Geometry check sheet. Reference: drawing and pictorial views, mm from the part's lowest x, y, z. Coordinates: 2 decimals unless noted, no trailing zeros. Loops run counter-clockwise (first coordinate to the right, second up) from the corner with the lowest first, then second, coordinate; pieces in that order, holes last. Notation, with made-up numbers: (-31, 82) - (18, 82) arc R20 cw to (18, 117) - close; hole circle Ø10 at (-36.5, -10). An arc over 180 degrees is marked (long way). One line per item, written item: value.
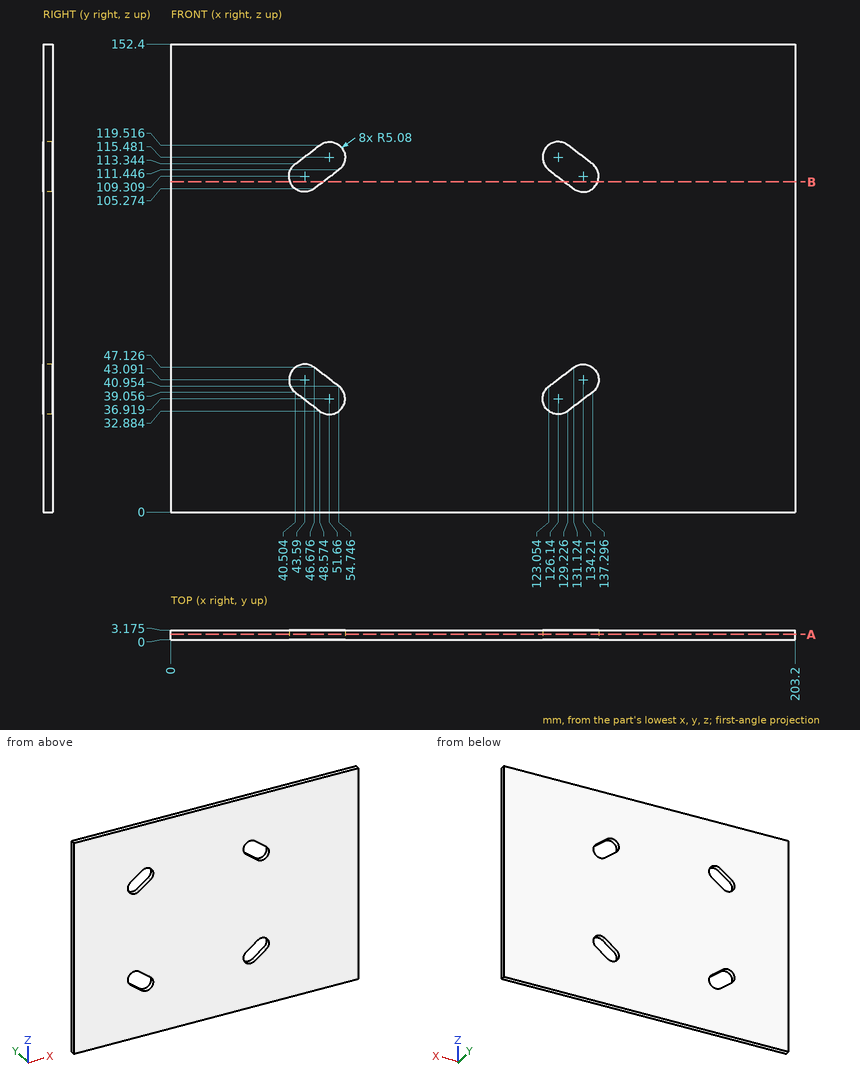
(1) Cross-section at A-A on y = 1.8. Record the cut outline in (x, z) (1 decimal), and give its area (3 significant figures).
Reply:
outline: (0, 0) - (203.2, 0) - (203.2, 152.4) - (0, 152.4) - close; hole (40.5, 39.1) - (48.6, 32.9) arc R5.1 ccw to (54.7, 41) - (46.7, 47.1) arc R5.1 ccw to start; hole (40.5, 113.3) arc R5.1 ccw to (46.7, 105.3) - (54.7, 111.4) arc R5.1 ccw to (48.6, 119.5) - close; hole (123.1, 41) arc R5.1 ccw to (129.2, 32.9) - (137.3, 39.1) arc R5.1 ccw to (131.1, 47.1) - close; hole (123.1, 111.4) - (131.1, 105.3) arc R5.1 ccw to (137.3, 113.3) - (129.2, 119.5) arc R5.1 ccw to start
area: 30,200 mm2
(2) Material ranges on probe 1 along X at (y, z) = (3, 110) (1 decimal); probe 2 along X at (y, z) = (0.9, 117) (1 decimal); probe 3 along Z at (x, y) = (53.5, 0.7) (1 decimal), recorded low to high. Write a range as from..to.
Reply:
probe 1: 0..38.6, 52.9..124.9, 139.2..203.2
probe 2: 0..45.3, 56.5..121.3, 132.5..203.2
probe 3: 0..32.2, 41.9..110.5, 120.2..152.4
(3) Cross-section at B-B on z = 107.5. Record the cut outline in (x, y) (1 decimal), and give its area (3 significant figures).
Reply:
outline: (0, 0) - (38.8, 0) - (38.8, 3.2) - (0, 3.2) - close; (49.6, 0) - (128.2, 0) - (128.2, 3.2) - (49.6, 3.2) - close; (139, 0) - (203.2, 0) - (203.2, 3.2) - (139, 3.2) - close
area: 577 mm2
